```python
from build123d import *


with BuildPart() as part:
    # Sketch → Revolution (revolve)
    with BuildSketch(Plane.YZ):
        Polygon((0, 39), (-6, 39), (-35, 10), (-35, 0), (-8, 0), (-1, 12.124356), (-1, 14.124356), (0, 15.124356), align=None)
    revolve(axis=Axis((0, 0, 0), (0, 0, 1)))


solid = part.part
```
Could you check a few things on this model? Use its own coordinates, in mm. A direction names the side the tool comes from. Round coordinates to 2 decimals unless told otherwise and drop trailing zeros. Loops run counter-clockwise (first coordinate to the right, second up) from the corner with the lowest first, then second, coordinate; pieces in that order, holes last. Notation, with made-up numbers: (64.25, 83.25) - (68.25, 83.25) arc R25 cw to (68.25, 101.25) - close; hole circle Ø10 at (66, -8). An arc over 180 degrees is marked (long way). Use CSV: the item, a comma, the result in double quotes.
Item 1: If we section it at A-A on z = 30.5: List the corners of the cut face in (x, y) for me.
Here are the results:
outline,"circle Ø29 at (0, 0)"
Item 2: If we mould it in two halves opening along X, with no side actions, what happens to faces 1 (the conical face through (-10.774, 2.392, 33.964)), 2 (the conical face through (-3.259, -1.695, 7.494)), 3 (the flat face through (0, 0, 39))? For each: pulls with the +X half, pulls with the -X half, needs draft (parallel to the pull), parting line crosses it, or undercut.
Here are the results:
face 1,"parting line crosses it"
face 2,"undercut"
face 3,"needs draft"
Item 3: If we section it at C-C on z = 35.5: List the corners of the cut face in (x, y) for me, then the cut area to 3 significant figures.
Here are the results:
outline,"circle Ø19 at (0, 0)"
area,"284 mm²"
Item 4: If we section it at B-B on z = 6: List the corners of the cut face in (x, y) for me, then the cut area to 3 significant figures.
Here are the results:
outline,"circle Ø70 at (0, 0); hole circle Ø9.07 at (0, 0)"
area,"3,780 mm²"
Item 5: For faces 4 (the flat face through (0.5, 8.3, 0)), 5 (the cylindrical face through (-1, 0, 13)), which set-ups out of +Z, -Z, +X, -X, +Y, -Y let a thin tool reach every point of the face, with its end or its side?
Here are the results:
face 4,"-Z, +X, -X, +Y, -Y"
face 5,"-Z"
Item 6: Will these pins go through, and if not, where does the flat tip stop? pin 1 (10 mm diameter, centred on y = 22, z = 21, fed in from +X); pin 2 (2 mm diameter, centred on y = 0, z = 22.5, fed in from -X); pin 3 (6 mm diameter, centred on x = -25, z = 16.5, fed in from +Y).
Here are the results:
pin 1,"stops at x = 20.58"
pin 2,"stops at x = -23.5"
pin 3,"stops at y = 20.41"
Item 7: I need wall thicknesses on L1, parallel to X at y = 0, z = 13; L2, parallel to Y at x = 0, z = 12; L3, parallel to Z at x = -13.5, y = -25. Which ranges of each line are inside material? Lowest first, please. Write a range as [from, to].
Here are the results:
L1,"x = [-32, -1], [1, 32]"
L2,"y = [-33, -1.07], [1.07, 33]"
L3,"z = [0, 16.59]"
